```python
from build123d import *

# Parameters (mm, degrees)
F1_DEPTH = 48
F3_DEPTH = 142.236757


with BuildPart() as f1:
    # F0 (on Top) → F1 (new body)
    with BuildSketch(Plane.XY):
        Polygon((0, 45), (-152.755526, 45), (-169.134186, 0), (0, 0), align=None)
        Polygon((0, 90), (0, 135), (-170, 135), (-271.362335, -207.913322), (-247.387787, -215), (-169.134186, 0), (-152.755526, 45), (-136.376865, 90), align=None)
    extrude(amount=F1_DEPTH)

    # F2 (on face) → F3 (cut, through all)
    with BuildSketch(Plane(origin=(-149.349245, 54.35868, 0), x_dir=(0.34202, 0.939693, 0), z_dir=(0.939693, -0.34202, 0))):
        Polygon((-286.64552, 24), (-57.847299, 48), (-286.64552, 48), align=None)
        Polygon((-306.842566, 24), (-286.64552, 24), (-286.64552, 48), (-315.660655, 48), align=None)
    extrude(amount=-F3_DEPTH, mode=Mode.SUBTRACT)

    # F4: F1 across plane


with BuildPart() as f1_1:
    add(f1.part)
    add(f1.part.mirror(Plane.YZ))


solid = f1_1.part
```
Build history of the part. All positions in model axes, mm. A direction names the side the tool comes from. Coordinates: 2 decimals unless noted, no trailing zeros. Write each loop counter-clockwise with the first axis right and the second up, starting at its lowest first coordinate (ties: lowest second). Pieces come first, ordered by that corner, then holes.
1. Drop flat-ended pins along their axis: pin 1 (4.5 mm diameter, centred on x = 257, y = -211.5, fed in from +Z); pin 2 (2 mm diameter, centred on y = 88, z = 31.5, fed in from -X); pin 3 (9.5 mm diameter, centred on x = -256, y = -209.5, fed in from +Z). Give the stop position or say it passes through.
Answer block:
pin 1: stops at z = 24.24
pin 2: stops at x = -184.19
pin 3: stops at z = 24.73
2. 3-axis set-ups, long thin cutter, end or side, ignore diameter. For faces 4 (the flat face through (-2, 45, 24)), 5 (the flat face through (2, 0, 24)), 6 (the flat face through (1, 13, 0)): which of +Z, -Z, +X, -X, +Y, -Y reach the whole face in a straight line?
Answer block:
face 4: +Z, -Z
face 5: +Z, -Z, -Y
face 6: -Z, +X, -X, +Y, -Y
3. Band-saw the part on B-B, the plane z = 14.5. Give the cut face in (x, y), and give its area (3 significant figures).
Answer block:
outline: (-271.36, -207.91) - (-247.39, -215) - (-169.13, 0) - (169.13, 0) - (247.39, -215) - (271.36, -207.91) - (170, 135) - (-170, 135) - close; hole (-152.76, 45) - (152.76, 45) - (136.38, 90) - (-136.38, 90) - close
area: 52,500 mm2
4. Band-saw the part on D-D, the plane z = 40.5. Give the cut face in (x, y).
Answer block:
outline: (-226.25, -55.3) - (-193.59, -67.19) - (-169.13, 0) - (169.13, 0) - (193.59, -67.19) - (226.25, -55.3) - (170, 135) - (-170, 135) - close; hole (-152.76, 45) - (152.76, 45) - (136.38, 90) - (-136.38, 90) - close
5. Drill centre lines: probe 1 along Y at (x, z) = (-69, 7.5); probe 2 along X at (y, z) = (-13, 3); probe 3 along X at (y, z) = (57, 15.5). Where is each one in solid material? Low to high.
Answer block:
probe 1: y = 0 to 45, 90 to 135
probe 2: x = -213.75 to -173.87, 173.87 to 213.75
probe 3: x = -193.06 to -148.39, 148.39 to 193.06
6. Band-saw the part on A-A, the plane x = 13. Give the cut face in (y, z), and give its area (3 significant figures).
Answer block:
outline: (0, 0) - (45, 0) - (45, 48) - (0, 48) - close; (90, 0) - (135, 0) - (135, 48) - (90, 48) - close
area: 4,320 mm2
7. Band-saw the part on C-C, the plane y = -126.5. Give the cut face in (x, z).
Answer block:
outline: (-247.3, 0) - (-215.18, 0) - (-215.18, 33.88) - (-247.3, 32.73) - close; (215.18, 0) - (247.3, 0) - (247.3, 32.73) - (215.18, 33.88) - close
8. Pull direction X, two halves, no side cores. Call faces 1 (the flat face through (-219.972, -34.056, 18.331)), 2 (the flat face through (219.972, -34.056, 18.331)), 3 (the flat face through (-144.681, 67.185, 23.664)): released by +X, released by -X, zero draft, split by the parting line, or undercut.
Answer block:
face 1: released by -X
face 2: released by +X
face 3: undercut
